```python
from build123d import *

# Parameters (mm, degrees)
SKETCH1_W           = 35
SKETCH1_H           = 0.7
SKETCH1_H_2         = 35
BOSS_EXTRUDE1_DEPTH = 2
CHAMFER1_SIZE       = 3
SKETCH4_R           = 2.6
SKETCH4_R_2         = 1.58
BOSS_EXTRUDE2_DEPTH = 1.5


with BuildPart() as part:
    # Sketch1 → Boss-Extrude1 (new body)
    with BuildSketch(Plane(origin=(0, 0, 0), x_dir=(1, 0, 0), z_dir=(0, 1, 0))):
        with BuildLine():
            Line((7.5, 17.5), (13.1, 17.5))
            Line((13.1, 17.5), (13.1, 30))
            Line((13.1, 30), (7.5, 30))
            Line((7.5, 30), (7.5, 25.524823935))
            ThreePointArc((7.5, 25.524823935), (8.018677324, 24.703939201), (8.2, 23.75))
            ThreePointArc((8.2, 23.75), (8.018677324, 22.796060799), (7.5, 21.975176065))
            Line((7.5, 21.975176065), (7.5, 17.5))
        make_face()
        with BuildLine():
            Line((-1.9, 30), (-1.9, 17.5))
            Line((-1.9, 17.5), (7.5, 17.5))
            Line((7.5, 17.5), (7.5, 21.975176065))
            ThreePointArc((7.5, 21.975176065), (3, 23.75), (7.5, 25.524823935))
            Line((7.5, 25.524823935), (7.5, 30))
            Line((7.5, 30), (-1.9, 30))
        make_face()
        with Locations((0, -17.85)):
            Rectangle(SKETCH1_W, SKETCH1_H)
        Rectangle(SKETCH1_W, SKETCH1_H_2)
    extrude(amount=BOSS_EXTRUDE1_DEPTH)

    # Chamfer1
    chamfer1_edges = [part.edges().sort_by_distance(p)[0] for p in [
        (-1.9, 1, -30),
        (13.1, 1, -30),
        (17.5, 1, -17.5),
        (17.5, 1, 18.2),
        (-17.5, 1, 18.2),
        (-17.5, 1, -17.5),
    ]]
    chamfer(chamfer1_edges, length=CHAMFER1_SIZE)

    # Sketch4 → Boss-Extrude2 (add)
    with BuildSketch(Plane(origin=(0, 2, 0), x_dir=(1, 0, 0), z_dir=(0, 1, 0))):
        with Locations((5.6, 23.75)):
            Circle(SKETCH4_R)
        with Locations((5.6, 23.75)):
            Circle(SKETCH4_R_2, mode=Mode.SUBTRACT)
    extrude(amount=-BOSS_EXTRUDE2_DEPTH)


solid = part.part
```
Geometry check sheet. Reference: the model listing, model coordinates, mm. A direction names the side the tool comes from. Round coordinates to 2 decimals unless told otherwise and drop trailing zeros. Loops run counter-clockwise (first coordinate to the right, second up) from the corner with the lowest first, then second, coordinate; pieces in that order, holes last. Notation, with made-up numbers: (-19.75, -25) -> (31.25, -25) arc R15 ccw to (31.25, -1) -> close; hole circle Ø2 at (-23, 37.25). An arc over 180 degrees is marked (long way). Use a Markdown table: item, result.
(1) Sectioned sample at B-B (y = 0.9). Enter the section's corners in (x, z).
Calculated:
| item | result |
|---|---|
| outline | (-17.5, -14.5) -> (-14.5, -17.5) -> (-1.9, -17.5) -> (-1.9, -27) -> (1.1, -30) -> (10.1, -30) -> (13.1, -27) -> (13.1, -17.5) -> (14.5, -17.5) -> (17.5, -14.5) -> (17.5, 15.2) -> (14.5, 18.2) -> (-14.5, 18.2) -> (-17.5, 15.2) -> close; hole circle Ø3.16 at (5.6, -23.75) |
(2) Sectioned sample at A-A (x = 5.6). Enter the section's corners in (y, z).
Calculated:
| item | result |
|---|---|
| outline | (0, -30) -> (2, -30) -> (2, -25.33) -> (0.5, -25.33) -> (0.5, -26.35) -> (0, -26.35) -> close; (0, -21.15) -> (0.5, -21.15) -> (0.5, -22.17) -> (2, -22.17) -> (2, 18.2) -> (0, 18.2) -> close |
(3) Mould release check, pull along X, two halves, no side actions. Record for faces 1 (the flat face through (6, 1, -30)), 2 (the flat face through (16, 1, 16.7)), 3 (the flat face through (6, 0.5, -22)): released by +X, released by -X, zero draft, split by the parting line, or undercut.
Calculated:
| item | result |
|---|---|
| face 1 | zero draft |
| face 2 | released by +X |
| face 3 | undercut |
(4) Sectioned sample at C-C (z = -18). Enter the section's corners in (x, y).
Calculated:
| item | result |
|---|---|
| outline | (-1.9, 0) -> (13.1, 0) -> (13.1, 2) -> (-1.9, 2) -> close |
(5) Set-up check for faces 4 (the flat face through (13.1, 1, -22)), 5 (the flat face through (17.5, 1, 1)), 6 (the flat face through (-8, 1, -17.5)): record each of +Z, -Z, +X, -X, +Y, -Y from which the full face is reachable in a straight line by a thin tool's end or side.
Calculated:
| item | result |
|---|---|
| face 4 | -Z, +X, +Y, -Y |
| face 5 | +Z, -Z, +X, +Y, -Y |
| face 6 | -Z, -X, +Y, -Y |
(6) Go/stop test with flat-tipped pins: P1, Ø0.7, axis at x = 13.5, y = 0.5, coming from the -Z side; P2, Ø3.5, axis at x = 5.6, z = -23.75, coming from the -Y side. Record where each tip stops, or that it passes through.
Calculated:
| item | result |
|---|---|
| P1 | z = -17.5 |
| P2 | y = 0.5 |
(7) Sectioned sample at D-D (x = 12.5). Enter the section's corners in (y, z), then the cut area to 3 significant figures.
Calculated:
| item | result |
|---|---|
| outline | (0, -27.6) -> (2, -27.6) -> (2, 18.2) -> (0, 18.2) -> close |
| area | 91.6 mm² |
(8) Scan lines: probe 1 along Z at (x, y) = (5.5, 0.1); probe 2 along X at (y, z) = (1.75, -23.75); probe 3 along Z at (x, y) = (5.6, 1.1). Record each from-to range of solid material in increasing order.
Calculated:
| item | result |
|---|---|
| probe 1 | -30 to -26.35, -21.15 to 18.2 |
| probe 2 | -1.9 to 4.02, 7.18 to 13.1 |
| probe 3 | -30 to -25.33, -22.17 to 18.2 |
